```python
from build123d import *

# Parameters (mm, degrees)
F0_W     = 122
F0_H     = 122
F0_R     = 2
F0_R_2   = 55
F0_H_2   = 1
F1_DEPTH = 2
F0_W_2   = 1
F2_DEPTH = 25
F3_DEPTH = 24
F4_DEPTH = 1
F5_W     = 23
F5_H     = 1
F6_DEPTH = 1
F7_W     = 23
F7_H     = 1
F8_DEPTH = 1


with BuildPart() as f1:
    # F0 (on Front) → F1 (new body)
    with BuildSketch(Plane.XZ):
        Rectangle(F0_W, F0_H)
        with Locations((-52.5, -52.5)):
            Circle(F0_R, mode=Mode.SUBTRACT)
        with Locations((52.5, -52.5)):
            Circle(F0_R, mode=Mode.SUBTRACT)
        with Locations((-52.5, 52.5)):
            Circle(F0_R, mode=Mode.SUBTRACT)
        Circle(F0_R_2, mode=Mode.SUBTRACT)
        with Locations((52.5, 52.5)):
            Circle(F0_R, mode=Mode.SUBTRACT)
        with Locations((0, 61.5)):
            Rectangle(F0_W, F0_H_2)
        with Locations((0, 62.5)):
            Rectangle(F0_W, F0_H_2)
    extrude(amount=F1_DEPTH)

    # F0 (on Front) → F2 (join)
    with BuildSketch(Plane.XZ):
        Polygon((61, 61), (61, -61), (-61, -61), (-61, 61), (-61, 62), (-62, 62), (-62, -62), (62, -62), (62, 62), (61, 62), align=None)
        with Locations((61.5, 62.5)):
            Rectangle(F0_W_2, F0_H_2)
        with Locations((-61.5, 62.5)):
            Rectangle(F0_W_2, F0_H_2)
    extrude(amount=F2_DEPTH)

    # F0 (on Front) → F3 (join)
    with BuildSketch(Plane.XZ):
        Polygon((62, 63), (62, 62), (62, -62), (-62, -62), (-62, 62), (-62, 63), (-63, 63), (-63, -63), (63, -63), (63, 63), align=None)
    extrude(amount=F3_DEPTH)

    # F0 (on Front) → F4 (cut)
    with BuildSketch(Plane.XZ):
        Polygon((62, 63), (62, 62), (62, -62), (-62, -62), (-62, 62), (-62, 63), (-63, 63), (-63, -63), (63, -63), (63, 63), align=None)
        with Locations((61.5, 62.5)):
            Rectangle(F0_W_2, F0_H_2)
        with Locations((0, 62.5)):
            Rectangle(F0_W, F0_H_2)
        with Locations((-61.5, 62.5)):
            Rectangle(F0_W_2, F0_H_2)
    extrude(amount=F4_DEPTH, mode=Mode.SUBTRACT)

    # F5 (on face) → F6 (join)
    with BuildSketch(Plane(origin=(-63, 0, 0), x_dir=(0, -1, 0), z_dir=(-1, 0, 0))):
        with Locations((12.5, 23.5)):
            Rectangle(F5_W, F5_H)
    extrude(amount=F6_DEPTH)

    # F7 (on face) → F8 (join)
    with BuildSketch(Plane.YZ.offset(63)):
        with Locations((-12.5, 23.5)):
            Rectangle(F7_W, F7_H)
    extrude(amount=F8_DEPTH)


solid = f1.part
```
The listing builds one solid part. Answer for the finished solid, in the listing's coordinates (mm). A direction names the side the tool comes from. Give positions to 0.01 mm unless a question says otherwise; leave off trailing zeros. Order: outer loops, then holes, each group sorted by start corner. A loop starts at its lowest first (then second) coordinate and runs counter-clockwise, first axis right, second up. Notation, with made-up numbers: (75, 11) -> (84, 11) arc R14 cw to (84, 16) -> close; hole circle Ø6 at (12.5, -22.75). An arc over 180 degrees is marked (long way). Answer as CSV lines item,"result". Start each with the question number.
Q1. A cutting plane is placed at B-B (x = -31). Determine the outline of the cut face in (y, z).
Q2. A cutting plane is placed at C-C (x = 52.5). Determine the outline of the cut face in (y, z), then the cut area to 3 significant figures.
Q3. Given pin 1 (1.5 mm diameter, centred on y = -17.5, z = -16, fed in from +X); pin 2 (0.8 mm diameter, centred on x = 19.5, y = -0.5, fed in from +Z); pin 3 (10 mm diameter, centred on y = -22.5, z = 30, fed in from -X), each flat-ended and moving along its own axis, determine where each tip first touches the part or whether it passes through.
Q4. Which of the six approach directions +Z, -Z, +X, -X, +Y, -Y give full straight-line access (tool end or side, diameter ignored) to faces 1 (the flat face through (-55, -2, 16)), 2 (the flat face through (-63, -12, 44)), 3 (the flat face through (63, -12, 43)), 4 (the flat face through (-63, -12, -19))?
Q5. A cutting plane is placed at A-A (z = 0). Determine the outline of the cut face in (x, y).
Q6. Find the intervals of material crossed by L1, parallel to X at y = -18.5, z = 22.5; L2, parallel to Y at x = 44, z = 46; L3, parallel to Z at x = -25, y = -23, in increasing order.
Q7. A cutting plane is placed at D-D (y = -14). Determine the outline of the cut face in (x, z).
Results found:
1,outline,"(-25, -62) -> (-24, -62) -> (-24, -63) -> (-1, -63) -> (-1, -62) -> (0, -62) -> (0, -45.43) -> (-2, -45.43) -> (-2, -61) -> (-25, -61) -> close; (-2, 45.43) -> (0, 45.43) -> (0, 62) -> (-1, 62) -> (-1, 63) -> (-2, 63) -> close"
2,outline,"(-25, -62) -> (-24, -62) -> (-24, -63) -> (-1, -63) -> (-1, -62) -> (0, -62) -> (0, -54.5) -> (-2, -54.5) -> (-2, -61) -> (-25, -61) -> close; (-2, -50.5) -> (0, -50.5) -> (0, -16.39) -> (-2, -16.39) -> close; (-2, 16.39) -> (0, 16.39) -> (0, 50.5) -> (-2, 50.5) -> close; (-2, 54.5) -> (0, 54.5) -> (0, 62) -> (-1, 62) -> (-1, 63) -> (-2, 63) -> close"
2,area,"213 mm2"
3,pin 1,"x = 63"
3,pin 2,"z = 62"
3,pin 3,"x = -63"
4,face 1,"+Z, -Y"
4,face 2,"+Z, -X, +Y, -Y"
4,face 3,"+Z, +X, +Y, -Y"
4,face 4,"-Z, -X, +Y, -Y"
5,outline,"(-63, -24) -> (-62, -24) -> (-62, -25) -> (-61, -25) -> (-61, -2) -> (-55, -2) -> (-55, 0) -> (-62, 0) -> (-62, -1) -> (-63, -1) -> close; (55, -2) -> (61, -2) -> (61, -25) -> (62, -25) -> (62, -24) -> (63, -24) -> (63, -1) -> (62, -1) -> (62, 0) -> (55, 0) -> close"
6,L1,"-63 to -61, 61 to 63"
6,L2,"-2 to 0"
6,L3,"-63 to -61"
7,outline,"(-64, 23) -> (-63, 23) -> (-63, -63) -> (63, -63) -> (63, 23) -> (64, 23) -> (64, 24) -> (63, 24) -> (63, 63) -> (61, 63) -> (61, -61) -> (-61, -61) -> (-61, 63) -> (-63, 63) -> (-63, 24) -> (-64, 24) -> close"
